from build123d import *

# Parameters (mm, degrees)
SKETCH1_R           = 7.5
BOSS_EXTRUDE1_DEPTH = 160
BOSS_EXTRUDE2_START = 35
SKETCH1_3_R         = 50
BOSS_EXTRUDE2_DEPTH = 5
BOSS_EXTRUDE3_START = 115
SKETCH1_4_R         = 50
SKETCH1_4_R_2       = 7.5
BOSS_EXTRUDE3_DEPTH = 5
CUT_EXTRUDE1_START  = -10
SKETCH2_R           = 7.5
SKETCH2_R_2         = 5
CUT_EXTRUDE1_DEPTH  = 10


with BuildPart() as part:
    # Sketch1 → Boss-Extrude1 (new body)
    with BuildSketch(Plane(origin=(0, 0, 0), x_dir=(1, 0, 0), z_dir=(0, 1, 0))):
        with Locations(Location((0, 0, 0), (0, 0, 270))):
            Circle(SKETCH1_R)
    extrude(amount=BOSS_EXTRUDE1_DEPTH)

    # Sketch1_3 → Boss-Extrude2 (add)
    with BuildSketch(Plane(origin=(0, 0, 0), x_dir=(1, 0, 0), z_dir=(0, 1, 0)).offset(BOSS_EXTRUDE2_START)):
        with Locations(Location((0, 0, 0), (0, 0, 270))):
            Circle(SKETCH1_3_R)
    extrude(amount=-BOSS_EXTRUDE2_DEPTH)

    # Sketch1_4 → Boss-Extrude3 (add)
    with BuildSketch(Plane(origin=(0, 0, 0), x_dir=(1, 0, 0), z_dir=(0, 1, 0)).offset(BOSS_EXTRUDE3_START)):
        with Locations(Location((0, 0, 0), (0, 0, 270))):
            Circle(SKETCH1_4_R)
        with Locations(Location((0, 0, 0), (0, 0, 270))):
            Circle(SKETCH1_4_R_2, mode=Mode.SUBTRACT)
    extrude(amount=BOSS_EXTRUDE3_DEPTH)

    # Sketch2 → Cut-Extrude1 (cut)
    with BuildSketch(Plane(origin=(0, 160, 0), x_dir=(1, 0, 0), z_dir=(0, 1, 0)).offset(CUT_EXTRUDE1_START)):
        with Locations(Location((0, 0, 0), (0, 0, 270))):
            Circle(SKETCH2_R)
        with Locations(Location((0, 0, 0), (0, 0, 270))):
            Circle(SKETCH2_R_2, mode=Mode.SUBTRACT)
    extrude(amount=CUT_EXTRUDE1_DEPTH, mode=Mode.SUBTRACT)


solid = part.part
For this review, take the finished solid that the model builds, in its own axes (mm). A direction names the side the tool comes from. Round coordinates to 2 decimals unless told otherwise and drop trailing zeros. Order: outer loops, then holes, each group sorted by start corner. A loop starts at its lowest first (then second) coordinate and runs counter-clockwise, first axis right, second up. Notation, with made-up numbers: (75.25, -36) -> (82.25, -36) arc R23 cw to (82.25, -15) -> close; hole circle Ø8 at (8, -26.5). An arc over 180 degrees is marked (long way). Write item = value, one per line. Start each with the question number.
1) Take a section at B-B on z = -28. State the section outline as (x, y) points, plus the area to 3 significant figures.
2) Take a section at A-A on x = 14. State the section outline as (y, z) points, plus the area to 3 significant figures.
3) The part is to be moulded in two halves that separate along Y. For faces 4 (the face through (-10, 120, -1)), 5 (the face through (0.33, 134.79, -7.493)), 6 (the face through (-10, 35, -1)), say which applies: +Y half, -Y half, draft (parallel to the pull), parting line (faces both ways), or undercut.
4) Insertion check: pin 1 (5 mm diameter, centred on x = 12, y = 65.5, fed in from -Z); pin 2 (5 mm diameter, centred on y = 83, z = -1.5, fed in from -X); pin 3 (5 mm diameter, centred on x = -11, z = -37.5, fed in from -Y); pin 4 (12 mm diameter, centred on y = 123, z = -10, fed in from +X). Each pin has a flat end and moves straight along its axis. Give the tip position at first contact, or say it passes through.
5) Take a section at C-C on x = 0. State the section outline as (y, z) points, plus the area to 3 significant figures.
6) Take a section at D-D on z = 0. State the section outline as (x, y) points.
7) To check wall thickness, follow line 1 (Y direction, x = 12, z = 7); line 2 (X direction, y = 99, z = 0.5); line 3 (Y direction, x = 7, z = -1.5). State the ranges of each line that lie inside material, in increasing order. Write a range as from..to.
8) Tool access review of faces 1 (the face through (0.33, 74.44, -7.493)), 2 (the face through (-5, 150, 2)), 3 (the face through (0.33, 14.79, -7.493)): name each direction out of +Z, -Z, +X, -X, +Y, -Y from which nothing blocks a thin tool from reaching the whole face with its end or side.
Verdict:
q1.outline = (-41.42, 30) -> (41.42, 30) -> (41.42, 35) -> (-41.42, 35) -> close; (-41.42, 115) -> (41.42, 115) -> (41.42, 120) -> (-41.42, 120) -> close
q1.area = 828 mm2
q2.outline = (30, -48) -> (35, -48) -> (35, 48) -> (30, 48) -> close; (115, -48) -> (120, -48) -> (120, 48) -> (115, 48) -> close
q2.area = 960 mm2
q3.face_4 = +Y half
q3.face_5 = draft
q3.face_6 = undercut
q4.pin_1 = through
q4.pin_2 = -7.5
q4.pin_3 = 30
q4.pin_4 = 49.77
q5.outline = (0, -7.5) -> (30, -7.5) -> (30, -50) -> (35, -50) -> (35, -7.5) -> (115, -7.5) -> (115, -50) -> (120, -50) -> (120, -7.5) -> (150, -7.5) -> (150, -5) -> (160, -5) -> (160, 5) -> (150, 5) -> (150, 7.5) -> (120, 7.5) -> (120, 50) -> (115, 50) -> (115, 7.5) -> (35, 7.5) -> (35, 50) -> (30, 50) -> (30, 7.5) -> (0, 7.5) -> close
q5.area = 3,200 mm2
q6.outline = (-50, 30) -> (-7.5, 30) -> (-7.5, 0) -> (7.5, 0) -> (7.5, 30) -> (50, 30) -> (50, 35) -> (7.5, 35) -> (7.5, 115) -> (50, 115) -> (50, 120) -> (7.5, 120) -> (7.5, 150) -> (5, 150) -> (5, 160) -> (-5, 160) -> (-5, 150) -> (-7.5, 150) -> (-7.5, 120) -> (-50, 120) -> (-50, 115) -> (-7.5, 115) -> (-7.5, 35) -> (-50, 35) -> close
q7.line_1 = 30..35, 115..120
q7.line_2 = -7.48..7.48
q7.line_3 = 0..150
q8.face_1 = none
q8.face_2 = +Y
q8.face_3 = -Y
